from build123d import *

# Parameters (mm, degrees)
F0_R     = 12.5
F0_R_2   = 10.2
F0_R_3   = 7.35
F1_DEPTH = 8
F2_DEPTH = 12.65
F3_DEPTH = 18.6
F4_R     = 10.175
F5_DEPTH = 6
F6_R     = 2.5
F7_R     = 2.5


with BuildPart() as f1:
    # F0 (on Top) → F1 (new body)
    with BuildSketch(Plane.XY):
        Circle(F0_R)
        Circle(F0_R_2, mode=Mode.SUBTRACT)
        Circle(F0_R_2)
        Circle(F0_R_3, mode=Mode.SUBTRACT)
        Circle(F0_R_3)
        with BuildLine():
            ThreePointArc((1.5, 5.4213121106), (5.5460137346, 0.9393384136), (3.2015621187, -4.625))
            Line((3.2015621187, -4.625), (-3.2015621187, -4.625))
            ThreePointArc((-3.2015621187, -4.625), (-5.5460137346, 0.9393384136), (-1.5, 5.4213121106))
            Line((-1.5, 5.4213121106), (-1.5, 4.625))
            Line((-1.5, 4.625), (1.5, 4.625))
            Line((1.5, 4.625), (1.5, 5.4213121106))
        make_face(mode=Mode.SUBTRACT)
    extrude(amount=F1_DEPTH)

    # F0 (on Top) → F2 (join)
    with BuildSketch(Plane.XY):
        Circle(F0_R_2)
        Circle(F0_R_3, mode=Mode.SUBTRACT)
        Circle(F0_R_3)
        with BuildLine():
            ThreePointArc((1.5, 5.4213121106), (5.5460137346, 0.9393384136), (3.2015621187, -4.625))
            Line((3.2015621187, -4.625), (-3.2015621187, -4.625))
            ThreePointArc((-3.2015621187, -4.625), (-5.5460137346, 0.9393384136), (-1.5, 5.4213121106))
            Line((-1.5, 5.4213121106), (-1.5, 4.625))
            Line((-1.5, 4.625), (1.5, 4.625))
            Line((1.5, 4.625), (1.5, 5.4213121106))
        make_face(mode=Mode.SUBTRACT)
    extrude(amount=F2_DEPTH)

    # F0 (on Top) → F3 (join)
    with BuildSketch(Plane.XY):
        Circle(F0_R_3)
        with BuildLine():
            ThreePointArc((1.5, 5.4213121106), (5.5460137346, 0.9393384136), (3.2015621187, -4.625))
            Line((3.2015621187, -4.625), (-3.2015621187, -4.625))
            ThreePointArc((-3.2015621187, -4.625), (-5.5460137346, 0.9393384136), (-1.5, 5.4213121106))
            Line((-1.5, 5.4213121106), (-1.5, 4.625))
            Line((-1.5, 4.625), (1.5, 4.625))
            Line((1.5, 4.625), (1.5, 5.4213121106))
        make_face(mode=Mode.SUBTRACT)
    extrude(amount=F3_DEPTH)

    # F4 (on face) → F5 (join)
    with BuildSketch(Plane.XY.offset(18.6)):
        Circle(F4_R)
    extrude(amount=F5_DEPTH)

    # F6
    f6_edges = [f1.edges().sort_by_distance(p)[0] for p in [
        (-7.35, 0, 12.65),
    ]]
    fillet(f6_edges, radius=F6_R)

    # F7
    f7_edges = [f1.edges().sort_by_distance(p)[0] for p in [
        (-7.35, 0, 18.6),
    ]]
    fillet(f7_edges, radius=F7_R)


solid = f1.part
Here's how the part is built. I have some questions about the finished solid (model axes, mm). A direction names the side the tool comes from. Coordinates: 2 decimals unless noted, no trailing zeros. Order: outer loops, then holes, each group sorted by start corner. A loop starts at its lowest first (then second) coordinate and runs counter-clockwise, first axis right, second up. Notation, with made-up numbers: (5, -22) - (48, -22) arc R12 ccw to (48, -18) - close; hole circle Ø8 at (37, -8.5). An arc over 180 degrees is marked (long way). Use CSV: the item, a comma, the result in double quotes. Start each with the question number.
1. Suppose I cut it at D-D on z = 16.75. List the corners of the cut face in (x, y) for me (3 decimals), then the cut area to 3 significant figures.
2. Please list where these lines run through material, in increasing order: line 1 (Z direction, x = 9.75, y = 2.25); line 2 (Z direction, x = 11, y = -3.25); line 3 (Y direction, x = 4.25, z = 2.75). Write a range as from..to.
3. If we mould it in two halves opening along Y, with no side actions, what happens to faces 1 (the face through (-10.2, 1.9, 8)), 2 (the face through (-1.593, -7.175, 15.618)), 3 (the face through (-5.56, 0.85, 9.17))? For each: +Y half, -Y half, draft (parallel to the pull), parting line (faces both ways), or undercut.
4. Suppose I cut it at B-B on x = 0. List the corners of the cut face in (y, z) for me (3 decimals), then the cut area to 3 significant figures.
5. Suppose I cut it at C-C on y = 0. List the corners of the cut face in (x, z) for me (3 decimals), then the cut area to 3 significant figures.
6. I'm going to push flat-ended pins straight in: pin 1 (1.9 mm diameter, centred on x = -0.5, z = 12, fed in from +Y); pin 2 (5 mm diameter, centred on x = 4.5, z = 3, fed in from -Y); pin 3 (8 mm diameter, centred on x = 4.5, z = 8, fed in from -Y). Where does each tip first touch, or does it pass through?
7. For faces 4 (the face through (-2.206, -9.933, 21.558)), 5 (the face through (-10, 1, 12.65)), 6 (the face through (0, -4.625, 9)), 7 (the face through (0, 0, 24.6)), which set-ups out of +Z, -Z, +X, -X, +Y, -Y let a thin tool reach every point of the face, with its end or its side?
8. Suppose I cut it at A-A on z = 12. List the corners of the cut face in (x, y) for me (3 decimals), then the cut area to 3 significant figures.
Output:
1,outline,"circle Ø14.872 at (0, 0); hole (-3.202, -4.625) - (3.202, -4.625) arc R5.625 ccw to (1.5, 5.421) - (1.5, 4.625) - (-1.5, 4.625) - (-1.5, 5.421) arc R5.625 ccw to start"
1,area,"81.5 mm2"
2,line 1,"z = 0..12.65, 18.6..24.6"
2,line 2,"z = 0..8"
2,line 3,"y = -11.76..-3.68, 3.68..11.76"
3,face 1,"draft"
3,face 2,"parting line"
3,face 3,"undercut"
4,outline,"(-12.5, 0) - (-4.625, 0) - (-4.625, 18.6) - (4.625, 18.6) - (4.625, 0) - (12.5, 0) - (12.5, 8) - (10.2, 8) - (10.2, 12.65) - (9.85, 12.65) arc R2.5 cw to (7.35, 15.15) - (7.35, 16.1) arc R2.5 cw to (9.85, 18.6) - (10.175, 18.6) - (10.175, 24.6) - (-10.175, 24.6) - (-10.175, 18.6) - (-9.85, 18.6) arc R2.5 cw to (-7.35, 16.1) - (-7.35, 15.15) arc R2.5 cw to (-9.85, 12.65) - (-10.2, 12.65) - (-10.2, 8) - (-12.5, 8) - close"
4,area,"338 mm2"
5,outline,"(-12.5, 0) - (-5.625, 0) - (-5.625, 18.6) - (5.625, 18.6) - (5.625, 0) - (12.5, 0) - (12.5, 8) - (10.2, 8) - (10.2, 12.65) - (9.85, 12.65) arc R2.5 cw to (7.35, 15.15) - (7.35, 16.1) arc R2.5 cw to (9.85, 18.6) - (10.175, 18.6) - (10.175, 24.6) - (-10.175, 24.6) - (-10.175, 18.6) - (-9.85, 18.6) arc R2.5 cw to (-7.35, 16.1) - (-7.35, 15.15) arc R2.5 cw to (-9.85, 12.65) - (-10.2, 12.65) - (-10.2, 8) - (-12.5, 8) - close"
5,area,"301 mm2"
6,pin 1,"stops at y = 10.2"
6,pin 2,"stops at y = -12.34"
6,pin 3,"stops at y = -12.49"
7,face 4,"+Z"
7,face 5,"none"
7,face 6,"-Z"
7,face 7,"+Z, +X, -X, +Y, -Y"
8,outline,"circle Ø20.4 at (0, 0); hole (-3.202, -4.625) - (3.202, -4.625) arc R5.625 ccw to (1.5, 5.421) - (1.5, 4.625) - (-1.5, 4.625) - (-1.5, 5.421) arc R5.625 ccw to start"
8,area,"235 mm2"
